The model under review builds one solid part; all positions refer to its coordinate system, in mm. Face numbers are marked on the shaded views. A direction names the side the tool comes from. Coordinates: 2 decimals unless noted, no trailing zeros. Write each loop counter-clockwise with the first axis right and the second up, starting at its lowest first coordinate (ties: lowest second). Pieces come first, ordered by that corner, then holes.
```python
from build123d import *

# Parameters (mm, degrees)
SKETCH1_W                   = 6.3
SKETCH1_H                   = 6.3
BOSS_EXTRUDE1_DEPTH         = 61.675
TAP_DRILL_FOR_M3X0_5_TAP1_D = 2.5
FILLET1_R                   = 2


with BuildPart() as part:
    # Sketch1 → Boss-Extrude1 (new body)
    with BuildSketch(Plane(origin=(0, 0, 0), x_dir=(1, 0, 0), z_dir=(0, 1, 0))):
        with BuildLine():
            ThreePointArc((0, -12.5), (5.550824366, -5.550824366), (12.5, 0))
            ThreePointArc((12.5, 0), (-8.838834765, 8.838834765), (0, -12.5))
        make_face()
        Rectangle(SKETCH1_W, SKETCH1_H, mode=Mode.SUBTRACT)
    extrude(amount=-BOSS_EXTRUDE1_DEPTH)

    # Tap Drill for M3x0.5 Tap1 (through all)
    with Locations(Plane(origin=(0, 0, -7.5), x_dir=(0, 0, 1), z_dir=(0, 1, 0))):
        with Locations((0, 0), (7.5, 7.5), (7.5, -7.5), (15, 0)):
            Hole(TAP_DRILL_FOR_M3X0_5_TAP1_D / 2)

    # Fillet1
    fillet1_edges = [part.edges().sort_by_distance(p)[0] for p in [
        (0, -30.8375, 12.5),
        (12.5, -30.8375, 0),
    ]]
    fillet(fillet1_edges, radius=FILLET1_R)


solid = part.part
```
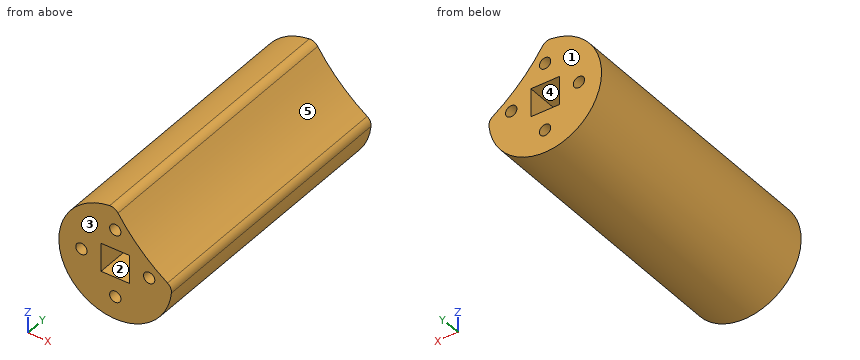
Item 1: Take a section at B-B, the plane x = -7.5. Write out the cut boundary in (y, z) (3 decimals).
Solved:
outline: (-61.675, -10) - (0, -10) - (0, -1.25) - (-61.675, -1.25) - close; (-61.675, 1.25) - (0, 1.25) - (0, 10) - (-61.675, 10) - close
Item 2: Mouldability with a two-part tool opening along Z and no side actions: class the marked faces 3, 4 and 5 as pulls with the +Z half, pulls with the -Z half, needs draft (parallel to the pull), parting line crosses it, or undercut.
Solved:
face 3: needs draft
face 4: undercut
face 5: pulls with the +Z half
Item 3: Take a section at D-D, the plane z = 5. Write out the cut boundary in (x, y) (3 decimals), plus the area to 3 significant figures.
Solved:
outline: (-11.456, -61.675) - (6.113, -61.675) - (6.113, 0) - (-11.456, 0) - close
area: 1,080 mm2
Item 4: Machinability: for the marked faces 1 and 2, which of the approach directions +Z, -Z, +X, -X, +Y, -Y give a long, thin tool a straight path to every point of the face, cutting with its end or side? Answer none if there is none.
Solved:
face 1: +Z, -Z, +X, -X, +Y
face 2: +Y, -Y
Item 5: Take a section at A-A, the plane z = -7.5. Write out the cut boundary in (x, y) (3 decimals).
Solved:
outline: (-10, -61.675) - (-1.25, -61.675) - (-1.25, 0) - (-10, 0) - close; (1.25, -61.675) - (10, -61.675) - (10, 0) - (1.25, 0) - close
Item 6: For pin 1 (1.5 mm diameter, centred on x = -9, y = -51, fed in from +Z); pin 2 (5 mm diameter, centred on y = -28, z = 4, fed in from +X); pin 3 (4 mm diameter, centred on x = 1.5, y = -55, fed in from +Z), all flat-tipped, find the tip position at first contact; note any pin that passes through.
Solved:
pin 1: stops at z = 9.39
pin 2: stops at x = 10.29
pin 3: stops at z = 12.37
Item 7: Take a section at C-C, the plane y = -52. Count the separate pieces of the cut face and the enclosed holes in it, plus the area to 3 significant figures.
Solved:
separate pieces: 1
enclosed holes: 5
area: 375 mm2
Item 8: To check wall thickness, follow line 1 along Z through (x, y) = (-1, -19.5); line 2 along X through (y, z) = (-12, 0); line 3 along X through (y, z) = (-17, 7.5). State the ranges of each line that lie inside material, in increasing order.
Solved:
line 1: z = -12.46 to -8.25, -6.75 to -3.15, 3.15 to 6.75, 8.25 to 12.45
line 2: x = -12.5 to -8.75, -6.25 to -3.15, 3.15 to 6.25, 8.75 to 12.15
line 3: x = -10 to -1.25, 1.25 to 3.73
